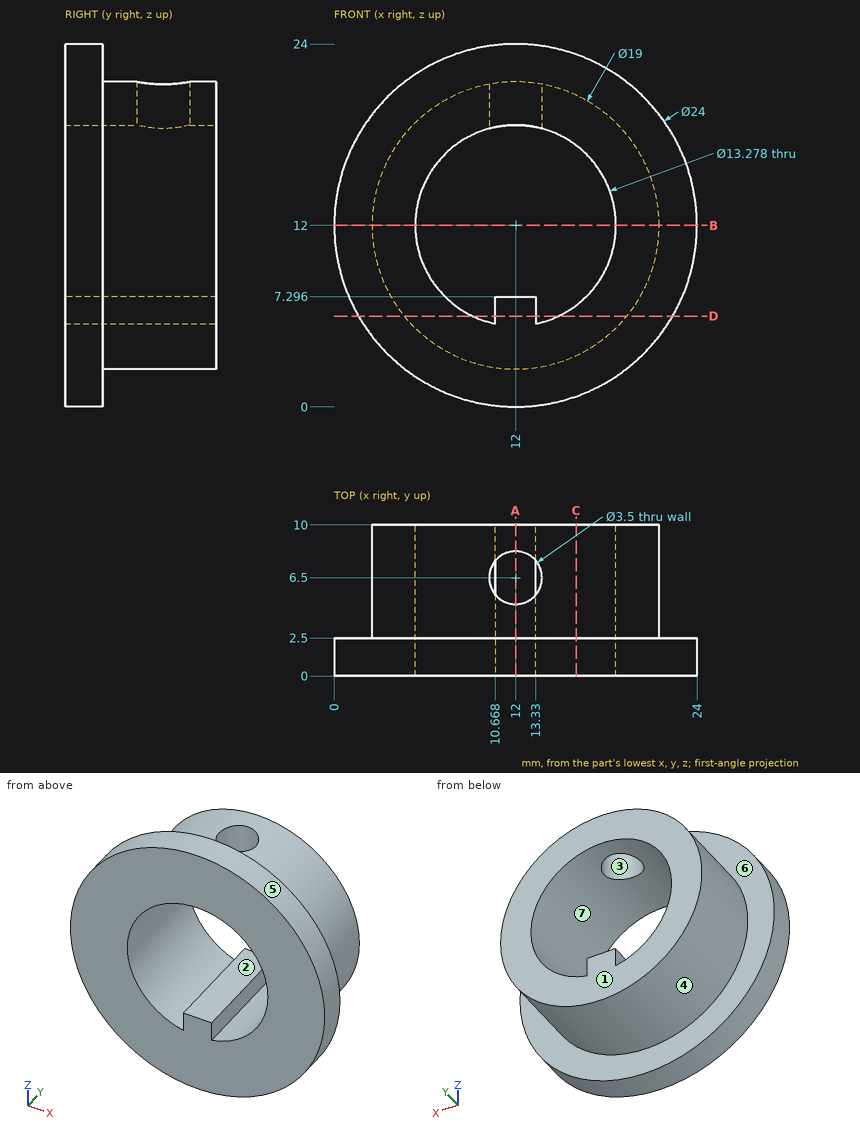
The figure shows three views and two pictorial views of one solid part (mm, origin at its lowest corner). Answer the questions. A direction names the side the tool comes from. Coordinates: 2 decimals unless noted, no trailing zeros. Write each loop counter-clockwise with the first axis right and the second up, starting at its lowest first coordinate (ties: lowest second). Pieces come first, ordered by that corner, then holes. Notation, with made-up numbers: (48.25, -23) -> (107.25, -23) arc R21 ccw to (107.25, -1) -> close; hole circle Ø1 at (72, 19). An arc over 180 degrees is marked (long way). Return JSON: item names as keys, results as strings.
(1) The part is cut by section C-C on x = 16. Give the vertices of the cut face in (y, z).
Answers below:
{"outline": "(0, 0.69) -> (2.5, 0.69) -> (2.5, 3.38) -> (10, 3.38) -> (10, 6.7) -> (0, 6.7) -> close; (0, 17.3) -> (10, 17.3) -> (10, 20.62) -> (2.5, 20.62) -> (2.5, 23.31) -> (0, 23.31) -> close"}
(2) The part is cut by section B-B on z = 12. Give the vertices of the cut face in (x, y), then the cut area to 3 significant figures.
Answers below:
{"outline": "(0, 0) -> (5.36, 0) -> (5.36, 10) -> (2.5, 10) -> (2.5, 2.5) -> (0, 2.5) -> close; (18.64, 0) -> (24, 0) -> (24, 2.5) -> (21.5, 2.5) -> (21.5, 10) -> (18.64, 10) -> close", "area": "69.7 mm^2"}
(3) Which of the six approach directions +Z, -Z, +X, -X, +Y, -Y give full straight-line access (tool end or side, diameter ignored) to the marked faces 1, 2, 3 and 4?
Answers below:
{"face 1": "+Z, -Z, +X, -X, +Y", "face 2": "+Y, -Y", "face 3": "+Z", "face 4": "+Y"}
(4) The part is cut by section A-A on x = 12. Give the vertices of the cut face in (y, z).
Answers below:
{"outline": "(0, 0) -> (2.5, 0) -> (2.5, 2.5) -> (10, 2.5) -> (10, 7.3) -> (0, 7.3) -> close; (0, 18.64) -> (4.75, 18.64) -> (4.75, 21.5) -> (2.5, 21.5) -> (2.5, 24) -> (0, 24) -> close; (8.25, 18.64) -> (10, 18.64) -> (10, 21.5) -> (8.25, 21.5) -> close"}
(5) For a pull along X with two mould halves and no side action, classify the marked faces 5, 6 and 7 as pulls with the +X half, pulls with the -X half, needs draft (parallel to the pull), parting line crosses it, or undercut.
Answers below:
{"face 5": "parting line crosses it", "face 6": "needs draft", "face 7": "undercut"}
(6) The part is cut by section D-D on z = 6. Give the vertices of the cut face in (x, y), then the cut area to 3 significant figures.
Answers below:
{"outline": "(1.61, 0) -> (9.16, 0) -> (9.16, 10) -> (4.63, 10) -> (4.63, 2.5) -> (1.61, 2.5) -> close; (10.67, 0) -> (13.33, 0) -> (13.33, 10) -> (10.67, 10) -> close; (14.84, 0) -> (22.39, 0) -> (22.39, 2.5) -> (19.37, 2.5) -> (19.37, 10) -> (14.84, 10) -> close", "area": "132 mm^2"}
(7) Each of these flat-tipped pins is pushed along its axis until it touches: P1, Ø0.5, axis at y = 5, z = 6.5, coming from the +X side; P2, Ø1.5, axis at y = 8, z = 6.5, coming from the -X side; P3, Ø0.8, axis at x = 12.5, y = 4.5, coming from the +Z side. Where does it stop, or does it pass through?
Answers below:
{"P1": "x = 19.92", "P2": "x = 3.77", "P3": "z = 21.5"}
(8) Consider line 1 along X through (y, z) = (2.75, 12); line 2 along Z through (x, y) = (12, 4); line 3 along Z through (x, y) = (11.75, 0.5). Determine where each line is inside the solid, lowest interval first. Write a range as from..to.
Answers below:
{"line 1": "2.5..5.36, 18.64..21.5", "line 2": "2.5..7.3, 18.64..21.5", "line 3": "0..7.3, 18.63..24"}
